```python
from build123d import *

# Parameters (mm, degrees)
BOSS_EXTRUDE2_DEPTH = 25.4
SKETCH3_R           = 4.7625
CUT_EXTRUDE1_DEPTH  = 36.576
CUT_EXTRUDE2_DEPTH  = 66.04
CUT_EXTRUDE3_DEPTH  = 2.032


with BuildPart() as part:
    # Sketch1 → Boss-Extrude2 (new body)
    with BuildSketch(Plane(origin=(-35.145897579, 0, 0), x_dir=(0, 0, -1), z_dir=(1, 0, 0))):
        Polygon((0, 0), (-19.05, 0), (-22.225, 0), (-22.225, 19.05), (-19.05, 19.05), (-19.05, 3.175), (0, 3.175), (0, 19.05), (3.175, 19.05), (3.175, 0), align=None)
    extrude(amount=BOSS_EXTRUDE2_DEPTH)

    # Sketch3 → Cut-Extrude1 (cut)
    with BuildSketch(Plane(origin=(0, 0, -3.175), x_dir=(-1, 0, 0), z_dir=(0, 0, -1))):
        with Locations((22.445897579, 11.3665)):
            Circle(SKETCH3_R)
    extrude(amount=-CUT_EXTRUDE1_DEPTH, mode=Mode.SUBTRACT)

    # Sketch4 → Cut-Extrude2 (cut)
    with BuildSketch(Plane(origin=(0, 3.175, 0), x_dir=(1, 0, 0), z_dir=(0, 1, 0))):
        with BuildLine():
            Line((-29.430897579, -2.54), (-15.460897579, -2.54))
            ThreePointArc((-15.460897579, -2.54), (-13.555897579, -4.445), (-15.460897579, -6.35))
            Line((-15.460897579, -6.35), (-29.430897579, -6.35))
            ThreePointArc((-29.430897579, -6.35), (-31.335897579, -4.445), (-29.430897579, -2.54))
        make_face()
    extrude(amount=-CUT_EXTRUDE2_DEPTH, mode=Mode.SUBTRACT)

    # Sketch7 → Cut-Extrude3 (cut)
    with BuildSketch(Plane(origin=(0, 3.175, 0), x_dir=(1, 0, 0), z_dir=(0, 1, 0))):
        with BuildLine():
            Line((-29.430897579, -1.27), (-15.460897579, -1.27))
            ThreePointArc((-15.460897579, -1.27), (-12.285897579, -4.445), (-15.460897579, -7.62))
            Line((-15.460897579, -7.62), (-29.430897579, -7.62))
            ThreePointArc((-29.430897579, -7.62), (-32.605897579, -4.445), (-29.430897579, -1.27))
        make_face()
    extrude(amount=-CUT_EXTRUDE3_DEPTH, mode=Mode.SUBTRACT)


solid = part.part
```
Model file for the job. Use its own axes, mm. A direction names the side the tool comes from. Round coordinates to 2 decimals unless told otherwise and drop trailing zeros. Write each loop counter-clockwise with the first axis right and the second up, starting at its lowest first coordinate (ties: lowest second). Pieces come first, ordered by that corner, then holes. Notation, with made-up numbers: (14, -33.5) - (65, -33.5) arc R22 ccw to (65, 5.5) - close; hole circle Ø3 at (3, 21.5). An arc over 180 degrees is marked (long way). Use CSV: the item, a comma, the result in double quotes. Start each with the question number.
Item 1: Tool access for faces 1 (the face through (-23, 3.175, 12)), 2 (the face through (-26.845, 9.542, 20.615)), 3 (the face through (-22, 2, 7.62)), 4 (the face through (-23, 19.05, -2)), 5 (the face through (-13.556, 0.58, 4.403)): list every direction of +Z, -Z, +X, -X, +Y, -Y with a clear straight run to the whole face (end or side of a thin tool).
Item 2: Band-saw the part on B-B (y = 2). Write the cut outline in (x, z) (3 decimals), and give its area (3 significant figures).
Item 3: Band-saw the part on D-D (y = 16.5). Write the cut outline in (x, z) (3 decimals), and give its area (3 significant figures).
Item 4: Pin check, flat tips, straight feed: P1, Ø8.5, axis at x = -22.45, y = 11.37, coming from the -Z side; P2, Ø2, axis at x = -21, z = 11.5, coming from the +Y side (3 decimals); P3, Ø5, axis at x = -24.5, z = 5.5, coming from the -Y side; P4, Ø3, axis at x = -27.5, z = 5.5, coming from the +Y side. Stop position of each tip, or through.
Item 5: Two-plate mould, pull along X, no slides. Class faces 6 (the face through (-25, 7, 0)), 7 (the face through (-35.146, 3, 11)), 8 (the face through (-26.845, 9.542, -1.61)): released by +X, released by -X, zero draft, split by the parting line, or undercut.
Item 6: Band-saw the part on A-A (x = -17). Write the cut outline in (y, z) (3 decimals).
Item 7: Band-saw the part on C-C (z = 5.25). Write the cut outline in (x, y) (3 decimals), and give its area (3 significant figures).
Item 8: Drill centre lines: L1, parallel to Z at x = -11, y = 8.75 (3 decimals); L2, parallel to Z at x = -22.75, y = 1.5 (3 decimals); L3, parallel to Y at x = -27.5, z = 12.5 (3 decimals). Where is each one in solid material? Low to high. Write a range as [from, to].
Checked values:
1,face 1,"+X, -X, +Y"
1,face 2,"+Z, -Z"
1,face 3,"+Y"
1,face 4,"+Z, -Z, +X, -X, +Y"
1,face 5,"+Y, -Y"
2,outline,"(-35.146, -3.175) - (-9.746, -3.175) - (-9.746, 22.225) - (-35.146, 22.225) - close; hole (-29.431, 1.27) - (-15.461, 1.27) arc R3.175 ccw to (-15.461, 7.62) - (-29.431, 7.62) arc R3.175 ccw to start"
2,area,"525 mm²"
3,outline,"(-35.146, -3.175) - (-9.746, -3.175) - (-9.746, 0) - (-35.146, 0) - close; (-35.146, 19.05) - (-9.746, 19.05) - (-9.746, 22.225) - (-35.146, 22.225) - close"
3,area,"161 mm²"
4,P1,"passes through"
4,P2,"stops at y = 3.175"
4,P3,"stops at y = 0"
4,P4,"stops at y = 1.14"
5,face 6,"zero draft"
5,face 7,"released by -X"
5,face 8,"undercut"
6,outline,"(0, -3.175) - (19.05, -3.175) - (19.05, 0) - (3.175, 0) - (3.175, 1.27) - (1.143, 1.27) - (1.143, 2.54) - (0, 2.54) - close; (0, 6.35) - (1.143, 6.35) - (1.143, 7.62) - (3.175, 7.62) - (3.175, 19.05) - (19.05, 19.05) - (19.05, 22.225) - (0, 22.225) - close"
7,outline,"(-35.146, 0) - (-31.157, 0) - (-31.157, 1.143) - (-32.502, 1.143) - (-32.502, 3.175) - (-35.146, 3.175) - close; (-13.734, 0) - (-9.746, 0) - (-9.746, 3.175) - (-12.39, 3.175) - (-12.39, 1.143) - (-13.734, 1.143) - close"
7,area,"19.9 mm²"
8,L1,"z = [-3.175, 0], [19.05, 22.225]"
8,L2,"z = [-3.175, 1.27], [7.62, 22.225]"
8,L3,"y = [0, 3.175]"
